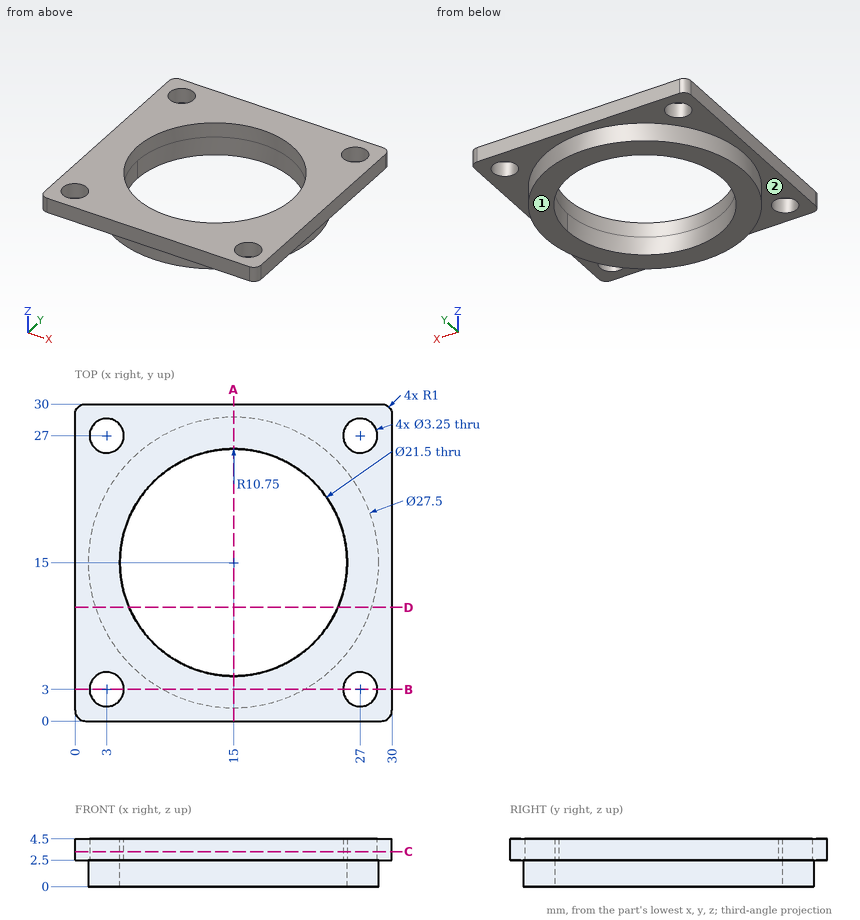
Answer from the drawing. Dimensions are ordinates in mm from the lowest x, y and z of the part. A direction names the side the tool comes from. Round coordinates to 2 decimals unless told otherwise and drop trailing zeros. Write each loop counter-clockwise with the first axis right and the second up, starting at its lowest first coordinate (ties: lowest second). Pieces come first, ordered by that corner, then holes.
1. The part is cut by section B-B, the plane y = 3. Determine the outline of the cut face in (x, z) (3 decimals).
2. Which of the six approach directions +Z, -Z, +X, -X, +Y, -Y give full straight-line access (tool end or side, diameter ignored) to the marked faces 1 and 2?
3. The part is cut by section C-C, the plane z = 3.3. Determine the outline of the cut face in (x, y) (3 decimals).
4. The part is cut by section A-A, the plane x = 15. Determine the outline of the cut face in (y, z), then the cut area to 3 significant figures.
5. The part is cut by section D-D, the plane y = 10.75. Determine the outline of the cut face in (x, z).
6. Straight lines are drawn through the part: L1, parallel to Y at x = 27, z = 3.6 (3 decimals); L2, parallel to Y at x = 2.5, z = 3; L3, parallel to Z at x = 11.25, y = 28.5. For each, find the intervals that lie inside material, in ascending order.
Values:
1. outline: (0, 2.5) - (1.375, 2.5) - (1.375, 4.5) - (0, 4.5) - close; (4.625, 2.5) - (8.287, 2.5) - (8.287, 0) - (21.713, 0) - (21.713, 2.5) - (25.375, 2.5) - (25.375, 4.5) - (4.625, 4.5) - close; (28.625, 2.5) - (30, 2.5) - (30, 4.5) - (28.625, 4.5) - close
2. face 1: -Z, +X, -X, +Y, -Y
2. face 2: -Z
3. outline: (0, 1) arc R1 ccw to (1, 0) - (29, 0) arc R1 ccw to (30, 1) - (30, 29) arc R1 ccw to (29, 30) - (1, 30) arc R1 ccw to (0, 29) - close; hole circle Ø3.25 at (3, 3); hole circle Ø3.25 at (3, 27); hole circle Ø21.5 at (15, 15); hole circle Ø3.25 at (27, 3); hole circle Ø3.25 at (27, 27)
4. outline: (0, 2.5) - (1.25, 2.5) - (1.25, 0) - (4.25, 0) - (4.25, 4.5) - (0, 4.5) - close; (25.75, 0) - (28.75, 0) - (28.75, 2.5) - (30, 2.5) - (30, 4.5) - (25.75, 4.5) - close
4. area: 32.0 mm2
5. outline: (0, 2.5) - (1.92, 2.5) - (1.92, 0) - (5.13, 0) - (5.13, 4.5) - (0, 4.5) - close; (24.87, 0) - (28.08, 0) - (28.08, 2.5) - (30, 2.5) - (30, 4.5) - (24.87, 4.5) - close
6. L1: y = 0 to 1.375, 4.625 to 25.375, 28.625 to 30
6. L2: y = 0 to 1.45, 4.55 to 25.45, 28.55 to 30
6. L3: z = 2.5 to 4.5
